from build123d import *

# Parameters (mm, degrees)
FILLET1_R = 0.5


with BuildPart() as part:
    # Sketch1 → Revolve1 (revolve)
    with BuildSketch(Plane.XY, mode=Mode.PRIVATE) as revolve1_sk:
        Polygon((-1.4605, 0), (-1.4605, 4), (0, 4), (0, 6), (-2.4605, 6), (-2.4605, 0), align=None)
    revolve(revolve1_sk.sketch.rotate(Axis((0, 0, 0), (0, -1, 0)), 270), axis=Axis((0, 0, 0), (0, -1, 0)))

    # Fillet1
    fillet1_edges = [part.edges().sort_by_distance(p)[0] for p in [
        (0, 0, -2.4605),
        (0, 6, -2.4605),
        (0, 0, -1.4605),
    ]]
    fillet(fillet1_edges, radius=FILLET1_R - 0.0001)  # a hair under: the kernel refuses the full size


solid = part.part
Model file for the job. Use its own axes, mm. Round coordinates to 2 decimals unless told otherwise and drop trailing zeros. Loops run counter-clockwise (first coordinate to the right, second up) from the corner with the lowest first, then second, coordinate; pieces in that order, holes last.
1. Drop flat-ended pins along their axis: P1, Ø1.5, axis at y = 1, z = -1, coming from the +X side; P2, Ø2.5, axis at x = 0, z = 0, coming from the -Y side; P3, Ø2.5, axis at x = -0.5, z = -0.5, coming from the -Y side. Give the stop position or say it passes through.
Check values:
P1: stops at x = 2.45
P2: stops at y = 4
P3: stops at y = 0
2. Wall check: probe 1 along X at (y, z) = (2.35, 0); probe 2 along Z at (x, y) = (-0.75, 0.9); probe 3 along Y at (x, z) = (0.3, 0). Give the ranges that are in metal, low to high.
Check values:
probe 1: x = -2.46 to -1.46, 1.46 to 2.46
probe 2: z = -2.34 to -1.25, 1.25 to 2.34
probe 3: y = 4 to 6
3. Band-saw the part on C-C, the plane y = 1.8. List the corners of the cut face in (x, z), and give its area (3 significant figures).
Check values:
outline: circle Ø4.92 at (0, 0); hole circle Ø2.92 at (0, 0)
area: 12.3 mm2
4. Band-saw the part on D-D, the plane y = 5.2. List the corners of the cut face in (x, z).
Check values:
outline: circle Ø4.92 at (0, 0)
5. Mould opens along Z. For faces 1 (the flat face through (0, 6, 0)), 2 (the flat face through (0, 4, 0)), 3 (the cylindrical face through (-0.739, 2.965, 2.347)) say: +Z half, -Z half, draft (parallel to the pull), parting line (faces both ways), or undercut.
Check values:
face 1: draft
face 2: undercut
face 3: parting line
